The drawing under review shows one solid part. Ordinate dimensions are in mm from its lowest x, y, z. Coordinates: 2 decimals unless noted, no trailing zeros. Write each loop counter-clockwise with the first axis right and the second up, starting at its lowest first coordinate (ties: lowest second). Pieces come first, ordered by that corner, then holes.
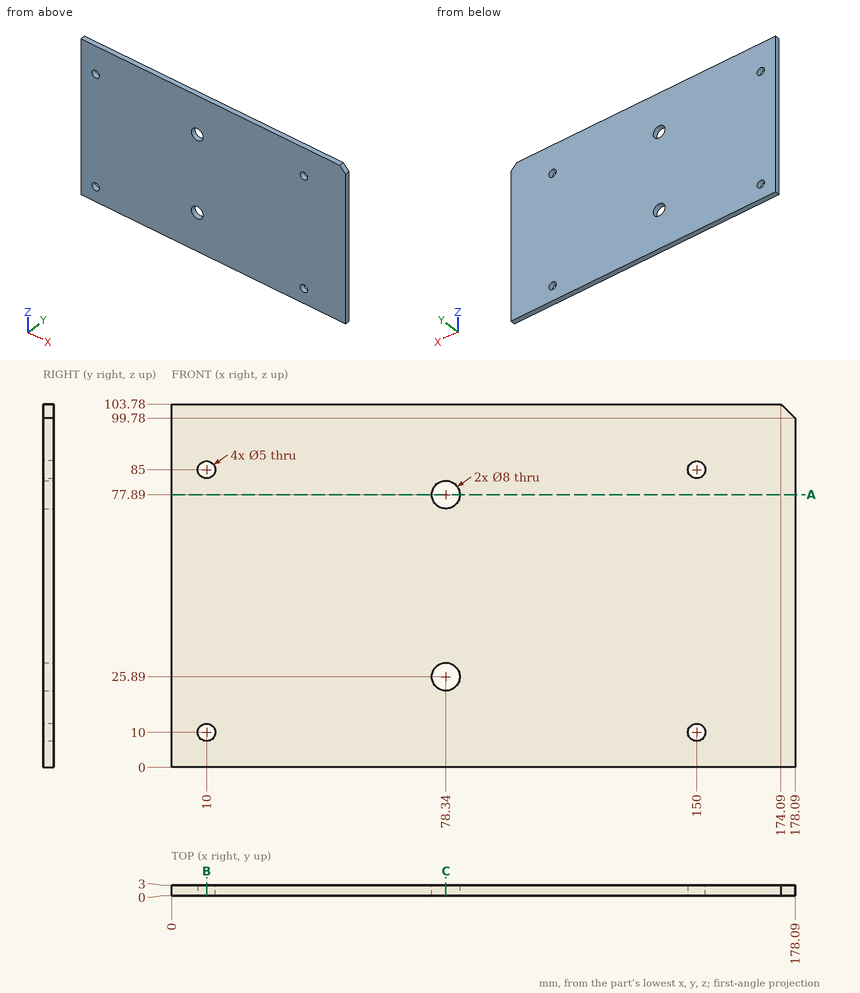
Q1. Add section A-A (z = 77.89). State the section outline as (x, y) points, then the cut area to 3 significant figures.
Ans:
outline: (0, 0) - (74.34, 0) - (74.34, 3) - (0, 3) - close; (82.34, 0) - (178.09, 0) - (178.09, 3) - (82.34, 3) - close
area: 510 mm2
Q2. For probe 1 along Z at (x, y) = (10, 2.35); probe 2 along X at (y, z) = (2.55, 10); probe 3 along X at (y, z) = (2.15, 77.89), list the stretches that pass through material, from the lowest coordinate up.
Ans:
probe 1: z = 0 to 7.5, 12.5 to 82.5, 87.5 to 103.78
probe 2: x = 0 to 7.5, 12.5 to 147.5, 152.5 to 178.09
probe 3: x = 0 to 74.34, 82.34 to 178.09
Q3. Add section B-B (x = 10). State the section outline as (y, z) points, then the cut area to 3 significant figures.
Ans:
outline: (0, 0) - (3, 0) - (3, 7.5) - (0, 7.5) - close; (0, 12.5) - (3, 12.5) - (3, 82.5) - (0, 82.5) - close; (0, 87.5) - (3, 87.5) - (3, 103.78) - (0, 103.78) - close
area: 281 mm2
Q4. Clearance check with a flat-ended pin moving along its axis: pin 1 Ø3 at (x, z) = (150, 85) entering from +Y. State where the tip first meets the part, or that it passes through.
Ans:
pin 1: passes through
Q5. Add section C-C (x = 78.34). State the section outline as (y, z) points.
Ans:
outline: (0, 0) - (3, 0) - (3, 21.89) - (0, 21.89) - close; (0, 29.89) - (3, 29.89) - (3, 73.89) - (0, 73.89) - close; (0, 81.89) - (3, 81.89) - (3, 103.78) - (0, 103.78) - close
